Design review of the part built by this model. Coordinates are the model's own, in mm. A direction names the side the tool comes from. Give positions to 0.01 mm unless a question says otherwise; leave off trailing zeros. Write each loop counter-clockwise with the first axis right and the second up, starting at its lowest first coordinate (ties: lowest second). Pieces come first, ordered by that corner, then holes. Notation, with made-up numbers: M 63,84 L 97,84 A19 ccw 97,89 Z; hole C 12,76 d9. An arc over 180 degrees is marked long. One line per item, written item: value. Start each with the question number.
```python
from build123d import *

# Parameters (mm, degrees)
F0_W     = 73.406
F0_H     = 25.4
F1_DEPTH = 14.224
F2_W     = 31.242
F2_H     = 25.4
F3_DEPTH = 28.575
F5_DEPTH = 22.099
F6_W     = 4.826
F6_H     = 11.049
F7_DEPTH = 104.649
F9_DEPTH = 26.925


# Not quite as in the source:
# - a pattern or mirror of a feature is missing from the dataset's text; its kind, count and spacing are read off the source's solid


with BuildPart() as f1:
    # F0 (on Front) → F1 (new body, symmetric)
    with BuildSketch(Plane.XZ):
        Rectangle(F0_W, F0_H)
    extrude(amount=F1_DEPTH, both=True)

    # F2 (on face) → F3 (join)
    with BuildSketch(Plane.XY.offset(12.7)):
        Polygon((-36.703, 7.874), (-36.703, -3.048), (-30.353, -3.048), (-30.353, -7.874), (32.893, -7.874), (32.893, -12.7), (36.703, -12.7), (36.703, 12.7), (32.893, 12.7), (32.893, 7.874), align=None)
        with Locations((52.324, 0)):
            Rectangle(F2_W, F2_H)
    f3 = extrude(amount=F3_DEPTH)

    # F3_copies: F3 across plane
    add(f3.mirror(Plane(origin=(0, 0, 0), x_dir=(-1, 0, 0), z_dir=(0, 0, -1))))

    # F4 (on face) → F5 (cut, through all)
    with BuildSketch(Plane.XZ.offset(7.874)):
        with BuildLine():
            ThreePointArc((-6.477, 35.814), (-12.065, 30.226), (-6.477, 24.638))
            Line((-6.477, 24.638), (17.399, 24.638))
            ThreePointArc((17.399, 24.638), (22.987, 30.226), (17.399, 35.814))
            Line((17.399, 35.814), (-6.477, 35.814))
        make_face()
    f5 = extrude(amount=-F5_DEPTH, mode=Mode.SUBTRACT)

    # F5_copies: F5 across plane
    add(f5.mirror(Plane(origin=(0, 0, 0), x_dir=(-1, 0, 0), z_dir=(0, 0, -1))), mode=Mode.SUBTRACT)

    # F6 (on face) → F7 (cut, through all)
    with BuildSketch(Plane.YZ.offset(67.945)):
        with Locations((-10.287, 18.2245)):
            Rectangle(F6_W, F6_H)
        with Locations((10.287, 18.2245)):
            Rectangle(F6_W, F6_H)
    f7 = extrude(amount=-F7_DEPTH, mode=Mode.SUBTRACT)

    # F7_copies: F7 across plane
    add(f7.mirror(Plane(origin=(0, 0, 0), x_dir=(-1, 0, 0), z_dir=(0, 0, -1))), mode=Mode.SUBTRACT)

    # F8 (on face) → F9 (cut, through all)
    with BuildSketch(Plane.XZ.offset(12.7)):
        Polygon((67.945, 41.275), (50.419, 23.749), (67.945, 23.749), align=None)
        Polygon((50.419, 23.749), (39.37, 12.7), (67.945, 12.7), (67.945, 23.749), align=None)
    f9 = extrude(amount=-F9_DEPTH, mode=Mode.SUBTRACT)

    # F9_copies: F9 across plane
    add(f9.mirror(Plane(origin=(0, 0, 0), x_dir=(-1, 0, 0), z_dir=(0, 0, -1))), mode=Mode.SUBTRACT)


solid = f1.part
```
Q1. For P1, Ø8, axis at y = -3, z = 6, coming from the +X side; P2, Ø10, axis at y = 10, z = 21, coming from the +X side; P3, Ø1.9, axis at x = -16, y = 11, coming from the -Z side, all flat-tipped, find the tip position at first contact; note any pin that passes through.
Q2. Take a section at C-C, the plane z = 26.5. Give the boundary of the cut face in (x, y).
Q3. Take a section at A-A, the plane y = 11.25. Give the boundary of the cut face in (x, z) (3 decimals), then the cut area to 3 significant figures.
Q4. The part is to be moulded in two halves that separate along X. For faces 1 (the face through (22.986, -0.11, -30.103)), 2 (the face through (46, -12.7, -32)), 3 (the face through (-12.064, -0.11, -30.349)), 4 (the face through (36.703, 0, 0)), say which applies: pulls with the +X half, pulls with the -X half, needs draft (parallel to the pull), parting line crosses it, or undercut.
Q5. Take a section at B-B, the plane x = -1.5. Give the boundary of the cut face in (y, z) (3 decimals), then the cut area to 3 significant figures.
Q6. Machinability: for faces 5 (the face through (42, 10, 23.749)), 6 (the face through (-34, -3.048, 27)), 7 (the face through (32.893, 10, 32)), which of the approach directions +Z, -Z, +X, -X, +Y, -Y give a long, thin tool a straight path to every point of the face, cutting with its end or side? Answer none if there is none.
Q7. Take a section at D-D, the plane y = 0.75. Give the boundary of the cut face in (x, z) (3 decimals), then the cut area to 3 significant figures.
Q8. Wall thickness on line 1 (Z direction, x = -1.5, y = -7) (3 decimals); line 2 (Z direction, x = 33.5, y = 8.5) (3 decimals); line 3 (Z direction, x = 39, y = 9.25) (3 decimals): over which ranges is each line inside the solid? List them lowest first. Write a range as from..to.
Results list:
1. P1: stops at x = 36.7
1. P2: stops at x = 52.67
1. P3: stops at z = -12.7
2. outline: M -36.7,-3.05 L -30.35,-3.05 L -30.35,-7.87 L -10.64,-7.87 L -10.64,7.87 L -36.7,7.87 Z; M 21.56,-7.87 L 32.89,-7.87 L 32.89,-12.7 L 53.17,-12.7 L 53.17,12.7 L 32.89,12.7 L 32.89,7.87 L 21.56,7.87 Z
3. outline: M -36.703,-12.7 L 36.703,-12.7 L 36.703,12.7 L -36.703,12.7 Z; M 32.893,-41.275 L 67.945,-41.275 L 50.419,-23.749 L 32.893,-23.749 Z; M 32.893,23.749 L 50.419,23.749 L 67.945,41.275 L 32.893,41.275 Z
3. area: 2,790 mm^2
4. face 1: undercut
4. face 2: needs draft
4. face 3: undercut
4. face 4: pulls with the +X half
5. outline: M -14.224,-12.7 L -7.874,-12.7 L -7.874,-24.638 L 7.874,-24.638 L 7.874,-12.7 L 14.224,-12.7 L 14.224,12.7 L 7.874,12.7 L 7.874,24.638 L -7.874,24.638 L -7.874,12.7 L -14.224,12.7 Z; M -7.874,-41.275 L 7.874,-41.275 L 7.874,-35.814 L -7.874,-35.814 Z; M -7.874,35.814 L 7.874,35.814 L 7.874,41.275 L -7.874,41.275 Z
5. area: 1,270 mm^2
6. face 5: +X, -X, +Y
6. face 6: +Z, -X, -Y
6. face 7: +Z, -X, +Y
7. outline: M -36.703,-41.275 L 67.945,-41.275 L 39.37,-12.7 L 36.703,-12.7 L 36.703,12.7 L 39.37,12.7 L 67.945,41.275 L -36.703,41.275 Z; hole M -6.477,-35.814 L 17.399,-35.814 A5.588 ccw 17.399,-24.638 L -6.477,-24.638 A5.588 ccw Z; hole M -6.477,24.638 L 17.399,24.638 A5.588 ccw 17.399,35.814 L -6.477,35.814 A5.588 ccw Z
7. area: 6,300 mm^2
8. line 1: z = -41.275..-35.814, -24.638..24.638, 35.814..41.275
8. line 2: z = -41.275..-23.749, -12.7..12.7, 23.749..41.275
8. line 3: z = -41.275..-23.749, 23.749..41.275
